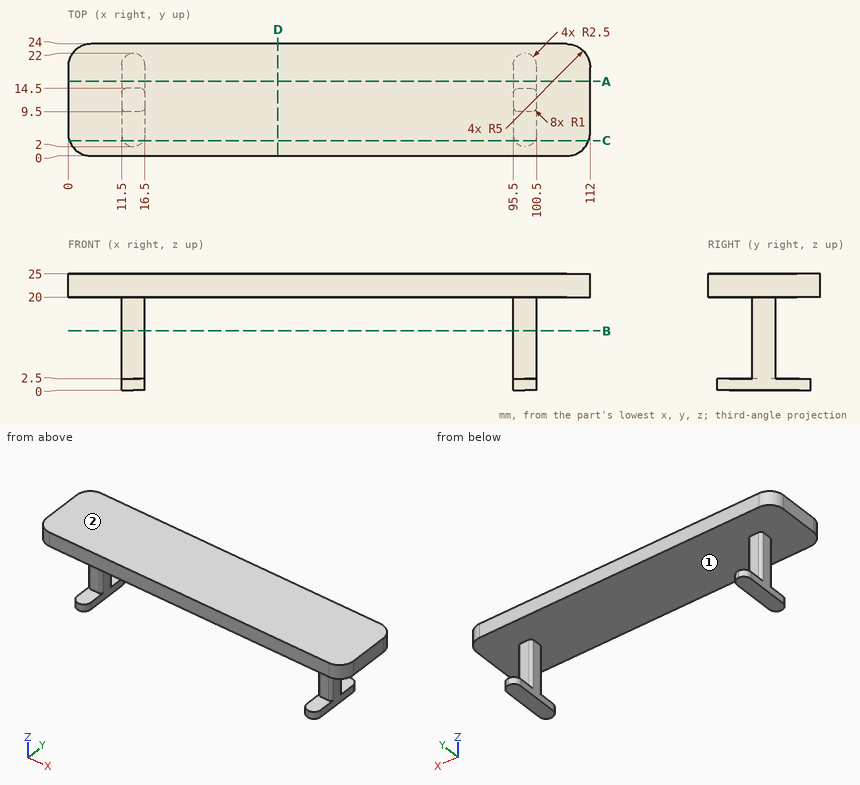
Study the drawing (mm; zero at the part's minimum x, y, z) and answer. Give positions to 0.01 mm unless a question says otherwise; leave off trailing zeros. Loops run counter-clockwise (first coordinate to the right, second up) from the corner with the lowest first, then second, coordinate; pieces in that order, holes last. Notation, with made-up numbers: (26, -1) - (31, -1) arc R25 ccw to (31, 30) - close; hole circle Ø4 at (17, 89). An arc over 180 degrees is marked (long way). Return JSON: item names as keys, results as strings. Group by question number.
1. Find section B-B (z = 12.75). Write down the section's boundary in (x, y).
2. Given pin 1 Ø6 at (x, z) = (12, 10.5) entering from -Y; pin 2 Ø12 at (y, z) = (9.5, 13) entering from +X; pin 3 Ø8 at (x, y) = (51.5, 5.5) entering from -Z, each flat-ended and moving along its own axis, determine where each tip first touches the part or whether it passes through.
3. Find section C-C (y = 3.25). Write down the section's boundary in (x, z).
4. Determine the mould class of the marked faces 1 and 2 for opening direction X: pulls with the +X half, pulls with the -X half, needs draft (parallel to the pull), parting line crosses it, or undercut.
5. Find section D-D (x = 45). Write down the section's boundary in (y, z), then the cut area to 3 significant figures.
6. Find section A-A (y = 16). Write down the section's boundary in (x, z), then the cut area to 3 significant figures.
7. Straight lines are drawn through the part: line 1 (X direction, y = 11.75, z = 5.5); line 2 (Z direction, x = 50, y = 6.25); line 3 (Y direction, x = 12.5, z = 15.5). For each, find the intervals that lie inside material, in ascending order. Write a range as [from, to].
Verdict:
{
 "1": {"outline": "(11.5, 10.5) arc R1 ccw to (12.5, 9.5) - (15.5, 9.5) arc R1 ccw to (16.5, 10.5) - (16.5, 13.5) arc R1 ccw to (15.5, 14.5) - (12.5, 14.5) arc R1 ccw to (11.5, 13.5) - close; (95.5, 10.5) arc R1 ccw to (96.5, 9.5) - (99.5, 9.5) arc R1 ccw to (100.5, 10.5) - (100.5, 13.5) arc R1 ccw to (99.5, 14.5) - (96.5, 14.5) arc R1 ccw to (95.5, 13.5) - close"},
 "2": {"pin 1": "stops at y = 9.5", "pin 2": "stops at x = 100.5", "pin 3": "stops at z = 20"},
 "3": {"outline": "(0.32, 20) - (111.68, 20) - (111.68, 25) - (0.32, 25) - close; (11.83, 0) - (16.17, 0) - (16.17, 2.5) - (11.83, 2.5) - close; (95.83, 0) - (100.17, 0) - (100.17, 2.5) - (95.83, 2.5) - close"},
 "4": {"face 1": "undercut", "face 2": "needs draft"},
 "5": {"outline": "(0, 20) - (24, 20) - (24, 25) - (0, 25) - close", "area": "120 mm^2"},
 "6": {"outline": "(0, 20) - (112, 20) - (112, 25) - (0, 25) - close; (11.5, 0) - (16.5, 0) - (16.5, 2.5) - (11.5, 2.5) - close; (95.5, 0) - (100.5, 0) - (100.5, 2.5) - (95.5, 2.5) - close", "area": "585 mm^2"},
 "7": {"line 1": "x = [11.5, 16.5], [95.5, 100.5]", "line 2": "z = [20, 25]", "line 3": "y = [9.5, 14.5]"}
}
